Design review of the part built by this model. Coordinates are the model's own, in mm. A direction names the side the tool comes from. Coordinates: 2 decimals unless noted, no trailing zeros. Write each loop counter-clockwise with the first axis right and the second up, starting at its lowest first coordinate (ties: lowest second). Pieces come first, ordered by that corner, then holes. Notation, with made-up numbers: M 24,-16.5 L 59,-16.5 A32 ccw 59,18.5 Z; hole C 62,-19 d9. An arc over 180 degrees is marked long. Write item = value, one per line.
Autodesk Inventor part; units mm, degrees
ref_plane "YZ Plane" through (0, 0, 0) normal (1, 0, 0) x (0, 1, 0)
ref_plane "XZ Plane" through (0, 0, 0) normal (0, 1, 0) x (-1, 0, 0)
ref_plane "XY Plane" through (0, 0, 0) normal (0, 0, 1) x (1, 0, 0)
sketch "Esquisse1" plane through (0, 0, 0) normal (0, 0, 1) x (1, 0, 0)
  circle A0 centre (0, 0) radius 3
  dimension "d0" = 6
extrude "Extrusion1" add sketch "Esquisse1" along normal blind 13.4
sketch "Esquisse2" plane through (0, 0, 13.4) normal (0, 0, 1) x (1, 0, 0)
  line L0 (-3, 3) -> (3, 3)
  line L1 (3, 3) -> (3, 1.5)
  line L2 (3, 1.5) -> (-3, 1.5)
  line L3 (-3, 1.5) -> (-3, 3)
  circle A0 centre (0, 0) radius 3
  dimension "d3" = 1.5
extrude "Extrusion2" cut sketch "Esquisse2" against normal blind 11.8 contours L0 A0 L2 L3 | L0 L1 L2 A0 | A0 L2 picked at (-0.7431, 1.6691)
sketch "Esquisse4" plane through (0, 0, 0) normal (0, 0, -1) x (-1, 0, 0)
  line L0 (-2.0616, 4) -> (2.0616, 4)
  line L1 (2.0616, -4) -> (-2.0616, -4)
  line L2 (0, -6.3) -> (0, 6.3) construction
  line L3 (6.3, 0) -> (-6.3, 0) construction
  arc A0 (2.0616, -4) -> (2.0616, 4) centre (0, 0) ccw
  arc A1 (-2.0616, 4) -> (-2.0616, -4) centre (0, 0) ccw
  dimension "d12" = 8
  dimension "d40" = 4.5
extrude "Extrusion4" add sketch "Esquisse4" along normal blind 5
sketch "Esquisse5" plane through (0, 0, -5) normal (0, 0, -1) x (-1, 0, 0)
  line L0 (6.5, 6.635) -> (-6.03, 6.635)
  line L1 (-6.03, 6.635) -> (-6.03, -6.635)
  line L2 (-6.03, -6.635) -> (6.5, -6.635)
  line L3 (6.5, -6.635) -> (6.5, 6.635)
  line L4 (9.006, 0) -> (-8.536, 0) construction
  line L5 (0, -9.289) -> (0, 9.289) construction
  point P0 (0, 0)
  dimension "d24" = 12.53
  dimension "d25" = 6.5
  dimension "d26" = 13.27
extrude "Extrusion5" add sketch "Esquisse5" along normal blind 7.5
chamfer "Chanfrein1" distance 0.75 distance2 1.68 1 edges at (0, 1.5, 13.4) measured on face at (-0.5642, -0.3597, 13.4)
chamfer "Chanfrein2" distance 0.75 distance2 1.68 2 edges at (2.9761, 0.378, 13.4) (-0.378, -2.9761, 13.4) measured on face at (-0.5788, -0.7991, 13.4)
thread "Filetage5"
thread "Filetage6"
properties part number "Potentiomètre"
Q1. Wall thickness on line 1 (Z direction, x = -1, y = 3.5); line 2 (Z direction, x = 4, y = -5.5); line 3 (Y direction, x = 0, z = 8.5): over which ranges is each line inside the solid? List them lowest first.
Check result:
line_1 = -12.5 to 0
line_2 = -12.5 to -5
line_3 = -3 to 1.5
Q2. Consider section A-A, the plane x = 0. State the section outline as (y, z) points (3 decimals).
Check result:
outline = M -6.635,-12.5 L 6.635,-12.5 L 6.635,-5 L 4,-5 L 4,0 L 3,0 L 3,1.6 L 1.5,1.6 L 1.5,11.72 L 0.75,13.4 L -2.25,13.4 L -3,11.72 L -3,0 L -4,0 L -4,-5 L -6.635,-5 Z
Q3. Consider section B-B, the plane z = 0.5. State the section outline as (x, y) points.
Check result:
outline = C 0,0 d6
Q4. Consider section D-D, the plane z = 6. State the section outline as (x, y) points, and give its area (3 significant figures).
Check result:
outline = M -2.6,1.5 A3 ccw long 2.6,1.5 Z
area = 22.7 mm²
Q5. For P1, Ø1.6, axis at x = -1, y = 2, coming from the +Z side; P2, Ø5, axis at y = 2.5, z = -0.5, coming from the -X side; P3, Ø4, axis at x = -2.5, y = 1, coming from the +Z side; P4, Ø4.5, axis at x = -0.5, z = -1.5, coming from the -Y side, all flat-tipped, find the tip position at first contact; note any pin that passes through.
Check result:
P1 = 12.39
P2 = -4.5
P3 = 13.4
P4 = -4
Q6. Machinability: for faces 1 (the flat face through (0, 4, -2)), 2 (the cylindrical face through (4.5, -0.1, -2.5)), 3 (the flat face through (0, -4, -2)), 4 (the cylindrical face through (-4.5, 0.1, -2.5)), which of the approach directions +Z, -Z, +X, -X, +Y, -Y give a long, thin tool a straight path to every point of the face, cutting with its end or side? Answer none if there is none.
Check result:
face_1 = +Z, +X, -X, +Y
face_2 = +Z, +X
face_3 = +Z, +X, -X, -Y
face_4 = +Z, -X
Q7. Consider section C-C, the plane x = -5.25. State the section outline as (y, z) points (3 decimals).
Check result:
outline = M -6.635,-12.5 L 6.635,-12.5 L 6.635,-5 L -6.635,-5 Z
